Build history of the part. All positions in model axes, mm. A direction names the side the tool comes from. Give positions to 0.01 mm unless a question says otherwise; leave off trailing zeros. Loops run counter-clockwise (first coordinate to the right, second up) from the corner with the lowest first, then second, coordinate; pieces in that order, holes last. Notation, with made-up numbers: (16, -16) -> (31, -16) arc R36 cw to (31, 19) -> close; hole circle Ø11 at (-14.5, 79.25). An arc over 180 degrees is marked (long way). Answer in a Markdown table with one row per item. Add a question column.
from build123d import *

# Parameters (mm, degrees)
SKETCH1_R           = 4.3
BOSS_EXTRUDE1_DEPTH = 3


with BuildPart() as part:
    # Sketch1 → Boss-Extrude1 (new body)
    with BuildSketch(Plane.XY):
        with BuildLine():
            Line((-35.59279418, 39.784944199), (-35.59279418, -39.784944199))
            Line((-35.59279418, -39.784944199), (35.59279418, -39.784944199))
            Line((35.59279418, -39.784944199), (35.59279418, 39.784944199))
            Line((35.59279418, 39.784944199), (10, 39.784944199))
            Line((10, 39.784944199), (10, 35.2))
            ThreePointArc((10, 35.2), (0, 25.2), (-10, 35.2))
            Line((-10, 35.2), (-10, 39.784944199))
            Line((-10, 39.784944199), (-35.59279418, 39.784944199))
        make_face()
        with Locations((-27.15, -30.3)):
            Circle(SKETCH1_R, mode=Mode.SUBTRACT)
        with Locations((27.15, -30.3)):
            Circle(SKETCH1_R, mode=Mode.SUBTRACT)
        with Locations((-27.15, 30.3)):
            Circle(SKETCH1_R, mode=Mode.SUBTRACT)
        with Locations((27.15, 30.3)):
            Circle(SKETCH1_R, mode=Mode.SUBTRACT)
    extrude(amount=BOSS_EXTRUDE1_DEPTH)


solid = part.part
(1) Flat gauge pins, fed straight in: pin 1 Ø12 at (x, y) = (-13, 8) entering from -Z; pin 2 Ø5 at (x, y) = (27.15, 30.3) entering from -Z. Where does each tip first touch, or does it go through?
(2) 3-axis set-ups, long thin cutter, end or side, ignore diameter. For faces 4 (the cylindrical face through (26.59, 34.563, 1.479)), 5 (the flat face through (10, 38, 1)): which of +Z, -Z, +X, -X, +Y, -Y reach the whole face in a straight line?
(3) Two-plate mould, pull along Y, no slides. Class faces 1 (the flat face through (0, -39.785, 1)), 2 (the flat face through (-10, 37, 1)), 3 (the cylindrical face through (-27.71, 34.563, 1.479)): released by +Y, released by -Y, zero draft, split by the parting line, or undercut.
(4) Saw through at B-B, the plane z = 1.1. List the corners of the cut face in (x, y), then the cut area to 3 significant figures.
(5) Saw through at D-D, the plane y = 30.3. List the corners of the cut face in (x, z).
(6) Saw through at A-A, the plane x = 27.15. List the corners of the cut face in (y, z).
(7) Saw through at C-C, the plane y = -30.3. List the corners of the cut face in (x, z), then the cut area to 3 significant figures.
(8) Wall check: line 1 along Y through (x, z) = (-27.15, 1.65); line 2 along X through (y, z) = (33.5, 0.85); line 3 along X through (y, z) = (-28, 1.4). Give the ranges that are in metal, low to high. Write a range as from..to.
Worked answers:
| question | item | result |
|---|---|---|
| 1 | pin 1 | z = 0 |
| 1 | pin 2 | through |
| 2 | face 4 | +Z, -Z |
| 2 | face 5 | +Z, -Z, +Y |
| 3 | face 1 | released by -Y |
| 3 | face 2 | zero draft |
| 3 | face 3 | undercut |
| 4 | outline | (-35.59, -39.78) -> (35.59, -39.78) -> (35.59, 39.78) -> (10, 39.78) -> (10, 35.2) arc R10 cw to (-10, 35.2) -> (-10, 39.78) -> (-35.59, 39.78) -> close; hole circle Ø8.6 at (-27.15, -30.3); hole circle Ø8.6 at (-27.15, 30.3); hole circle Ø8.6 at (27.15, -30.3); hole circle Ø8.6 at (27.15, 30.3) |
| 4 | area | 5,180 mm^2 |
| 5 | outline | (-35.59, 0) -> (-31.45, 0) -> (-31.45, 3) -> (-35.59, 3) -> close; (-22.85, 0) -> (-8.72, 0) -> (-8.72, 3) -> (-22.85, 3) -> close; (8.72, 0) -> (22.85, 0) -> (22.85, 3) -> (8.72, 3) -> close; (31.45, 0) -> (35.59, 0) -> (35.59, 3) -> (31.45, 3) -> close |
| 6 | outline | (-39.78, 0) -> (-34.6, 0) -> (-34.6, 3) -> (-39.78, 3) -> close; (-26, 0) -> (26, 0) -> (26, 3) -> (-26, 3) -> close; (34.6, 0) -> (39.78, 0) -> (39.78, 3) -> (34.6, 3) -> close |
| 7 | outline | (-35.59, 0) -> (-31.45, 0) -> (-31.45, 3) -> (-35.59, 3) -> close; (-22.85, 0) -> (22.85, 0) -> (22.85, 3) -> (-22.85, 3) -> close; (31.45, 0) -> (35.59, 0) -> (35.59, 3) -> (31.45, 3) -> close |
| 7 | area | 162 mm^2 |
| 8 | line 1 | -39.78..-34.6, -26..26, 34.6..39.78 |
| 8 | line 2 | -35.59..-30.02, -24.28..-9.85, 9.85..24.28, 30.02..35.59 |
| 8 | line 3 | -35.59..-30.78, -23.52..23.52, 30.78..35.59 |
